Here's how the part is built. I have some questions about the finished solid (model axes, mm). A direction names the side the tool comes from. Coordinates: 2 decimals unless noted, no trailing zeros. Order: outer loops, then holes, each group sorted by start corner. A loop starts at its lowest first (then second) coordinate and runs counter-clockwise, first axis right, second up. Notation, with made-up numbers: (50, 3.25) - (102, 3.25) arc R31 cw to (102, 30.25) - close; hole circle Ø5 at (10.25, 89.5). An arc over 180 degrees is marked (long way). Answer as CSV lines item,"result". Start each with the question number.
Q1. For pin 1 Ø1.5 at (x, z) = (31, 4.5) entering from +Y; pin 2 Ø1.5 at (y, z) = (11, -0.5) entering from +X; pin 3 Ø8 at (x, z) = (5, -4.5) entering from +Y; pin 4 Ø4 at (x, y) = (13.5, 8.5) entering from +Z, each with a flat end and sliding along its axis, tell me the tip position at first contact or that it passes through.
Q2. For faces 1 (the face through (5, 5, 0)), 2 (the face through (6, 3, -10)), which set-ups out of +Z, -Z, +X, -X, +Y, -Y let a thin tool reach every point of the face, with its end or its side?
Q3. Suppose I cut it at A-A (z = 2.5). Please give me the cut outline in (x, y), then the cut area to 3 significant figures.
Q4. Thinking about a two-plate mould opening in X: for faces 3 (the face through (11.136, 3.646, 0.14)), 4 (the face through (7, 0, 0)), 5 (the face through (0, 2, 0)), 6 (the face through (24.59, 10.62, 4.97)), which applies, released by +X, released by -X, zero draft, split by the parting line, or undercut?
Q5. Suppose I cut it at B-B (x = 3.5). Please give me the cut outline in (y, z), then the cut area to 3 significant figures.
Q6. Suppose I cut it at C-C (z = -6.75). Please give me the cut outline in (x, y), then the cut area to 3 significant figures.
Q7. I need wall thicknesses on line 1 (X direction, y = 4.5, z = -3.5); line 2 (Y direction, x = 9, z = 6.5); line 3 (X direction, y = 4, z = 5.5). Which ranges of each line are inside material? Lowest first, please.
from build123d import *

# Parameters (mm, degrees)
BOSS_EXTRUDE2_DEPTH = 10
BOSS_EXTRUDE4_DEPTH = 30


with BuildPart() as part:
    # Sketch3 → Boss-Extrude2 (new, symmetric)
    with BuildSketch(Plane.XY):
        Polygon((0, 0), (0, 5), (10, 5), (14.195498156, 0), align=None)
    extrude(amount=BOSS_EXTRUDE2_DEPTH, both=True)

    # Sketch5 → Boss-Extrude4 (add)
    with BuildSketch(Plane(origin=(8.330260271, 6.989918321, 0), x_dir=(0, 0, -1), z_dir=(0.7660444431189745, 0.6427876096865437, 0))):
        with BuildLine():
            Line((-4, -9.124690328), (-5.963533203, -6.179390524))
            ThreePointArc((-5.963533203, -6.179390524), (-6.013157507, -5.152832402), (-5.131482908, -4.624690328))
            Line((-5.131482908, -4.624690328), (5.131482908, -4.624690328))
            ThreePointArc((5.131482908, -4.624690328), (6.013157507, -5.152832402), (5.963533203, -6.179390524))
            Line((5.963533203, -6.179390524), (4, -9.124690328))
            Line((4, -9.124690328), (-4, -9.124690328))
        make_face()
    extrude(amount=BOSS_EXTRUDE4_DEPTH)


solid = part.part
Here are the results:
1,pin 1,"stops at y = 20.6"
1,pin 2,"stops at x = 28.2"
1,pin 3,"stops at y = 5"
1,pin 4,"passes through"
2,face 1,"+Z, -Z, -X, +Y"
2,face 2,"-Z, +X, -X, +Y, -Y"
3,outline,"(0, 0) - (14.2, 0) - (37.18, 19.28) - (34.28, 22.73) - (11.3, 3.45) - (10, 5) - (0, 5) - close"
3,area,"195 mm²"
4,face 3,"undercut"
4,face 4,"zero draft"
4,face 5,"released by -X"
4,face 6,"released by +X"
5,outline,"(0, -10) - (5, -10) - (5, 10) - (0, 10) - close"
5,area,"100 mm²"
6,outline,"(0, 0) - (14.2, 0) - (10, 5) - (0, 5) - close"
6,area,"60.5 mm²"
7,line 1,"x = 0 to 10.42, 12.56 to 19.56"
7,line 2,"y = 0 to 5"
7,line 3,"x = 0 to 10.84, 12.07 to 15.46"
